The listing builds one solid part. Answer for the finished solid, in the listing's coordinates (mm). Round coordinates to 2 decimals unless told otherwise and drop trailing zeros. Write each loop counter-clockwise with the first axis right and the second up, starting at its lowest first coordinate (ties: lowest second). Pieces come first, ordered by that corner, then holes. Notation, with made-up numbers: (-1.75, 50.5) - (47.25, 50.5) arc R16 cw to (47.25, 69.5) - close; hole circle Ø5 at (35, -29). An arc over 180 degrees is marked (long way). Return JSON: item names as keys, results as strings. Group by question number.
from build123d import *

# Parameters (mm, degrees)
SKETCH1_W           = 13.843
SKETCH1_H           = 3.048
SKETCH1_W_2         = 3.175
SKETCH1_H_2         = 0.381
BOSS_EXTRUDE1_DEPTH = 3.048


with BuildPart() as part:
    # Sketch1 → Boss-Extrude1 (new body)
    with BuildSketch(Plane.XY):
        Polygon((-3.175, 6.731), (0, 6.731), (0, 53.213), (-3.175, 53.213), (-3.175, 64.77), (0, 64.77), (0, 68.834), (-22.098, 68.834), (-22.098, 63.754), (-25.273, 63.754), (-25.273, 3.2766), (-22.098, 3.2766), (-22.098, -3.048), (-19.558, -3.048), (-19.558, 0), (-5.715, 0), (-5.715, -3.048), (-3.175, -3.048), (-3.175, 6.35), align=None)
        with Locations((-12.6365, 66.294)):
            Rectangle(SKETCH1_W, SKETCH1_H, mode=Mode.SUBTRACT)
        with Locations((-1.5875, 6.5405)):
            Rectangle(SKETCH1_W_2, SKETCH1_H_2)
    extrude(amount=BOSS_EXTRUDE1_DEPTH)


solid = part.part
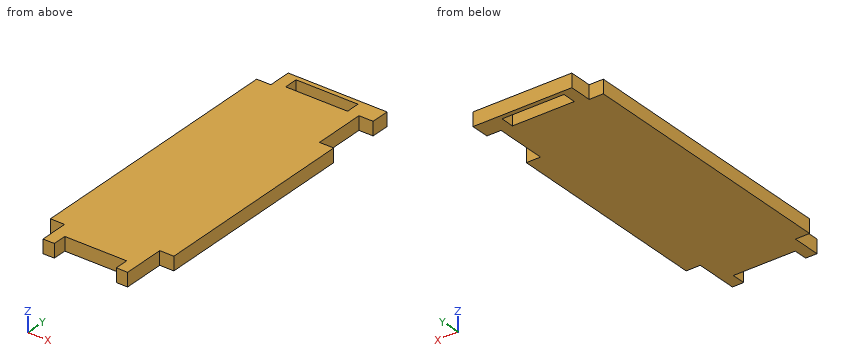
(1) Find section A-A (x = -15.5). Write down the section's boundary in (y, z), plus the area to 3 significant figures.
(2) Consider line 1 (Y direction, x = -13.25, z = 2.7); line 2 (X direction, y = 2.5, z = 2.6) (3 decimals); line 3 (X direction, y = 59, z = 2.15) (3 decimals). Determine where each line is inside the solid, lowest interval first.
(3) Find section C-C (y = 55). Write down the section's boundary in (x, z) (3 decimals), plus the area to 3 significant figures.
(4) Flat-ended cylindrical pins translate along their axes: pin 1 (1.5 mm diameter, centred on x = -7.5, z = 2, fed in from -Y); pin 2 (2 mm diameter, centred on x = -19.5, y = 24.5, fed in from -Z); pin 3 (1.5 mm diameter, centred on x = -2, z = 1, fed in from -Y); pin 4 (1.5 mm diameter, centred on y = -0.5, z = 1, fed in from +X) (3 decimals). Find the tip coordinate at first contact, or state that the pin passes through.
(5) Find section B-B (z = 1.4). Write down the section's boundary in (x, y) (3 decimals).
Check sheet entries:
{
 "1": {"outline": "(0, 0) - (64.77, 0) - (64.77, 3.05) - (0, 3.05) - close; (67.82, 0) - (68.83, 0) - (68.83, 3.05) - (67.82, 3.05) - close", "area": "201 mm^2"},
 "2": {"line 1": "y = 0 to 64.77, 67.82 to 68.83", "line 2": "x = -22.098 to -3.175", "line 3": "x = -25.273 to -3.175"},
 "3": {"outline": "(-25.273, 0) - (-3.175, 0) - (-3.175, 3.048) - (-25.273, 3.048) - close", "area": "67.4 mm^2"},
 "4": {"pin 1": "stops at y = 0", "pin 2": "stops at z = 0", "pin 3": "stops at y = 6.35", "pin 4": "stops at x = -3.175"},
 "5": {"outline": "(-25.273, 3.277) - (-22.098, 3.277) - (-22.098, -3.048) - (-19.558, -3.048) - (-19.558, 0) - (-5.715, 0) - (-5.715, -3.048) - (-3.175, -3.048) - (-3.175, 6.35) - (0, 6.35) - (0, 53.213) - (-3.175, 53.213) - (-3.175, 64.77) - (0, 64.77) - (0, 68.834) - (-22.098, 68.834) - (-22.098, 63.754) - (-25.273, 63.754) - close; hole (-19.558, 64.77) - (-5.715, 64.77) - (-5.715, 67.818) - (-19.558, 67.818) - close"}
}
